Geometry check sheet. Reference: the model listing, model coordinates, mm. A direction names the side the tool comes from. Round coordinates to 2 decimals unless told otherwise and drop trailing zeros. Order: outer loops, then holes, each group sorted by start corner. A loop starts at its lowest first (then second) coordinate and runs counter-clockwise, first axis right, second up.
```python
from build123d import *

# Parameters (mm, degrees)
ESBO_O1_W                                            = 500
ESBO_O1_H                                            = 200
RESSALTO_EXTRUS_O1_DEPTH                             = 40
REBAIXO_PARA_PARAFUSO_ALLEN_SEXTAVADO_DE_D           = 11
REBAIXO_PARA_PARAFUSO_ALLEN_SEXTAVADO_DE_DEPTH       = 40
REBAIXO_PARA_PARAFUSO_ALLEN_SEXTAVADO_DE_CBORE_D     = 18
REBAIXO_PARA_PARAFUSO_ALLEN_SEXTAVADO_DE_CBORE_DEPTH = 7.1
FURO_ROSCADO_DE_M18X2_0_D                            = 16
FURO_ROSCADO_DE_M18X2_0_DEPTH                        = 40


with BuildPart() as part:
    # Esboço1 → Ressalto-extrusão1 (new body)
    with BuildSketch(Plane(origin=(0, 0, 0), x_dir=(1, 0, 0), z_dir=(0, 1, 0))):
        Rectangle(ESBO_O1_W, ESBO_O1_H)
    extrude(amount=RESSALTO_EXTRUS_O1_DEPTH)

    # Rebaixo para parafuso Allen sextavado de M101
    with Locations(Plane(origin=(0, 40, 0), x_dir=(1, 0, 0), z_dir=(0, 1, 0))):
        with Locations((-225, 75), (-75, 75), (75, 75), (-75, -75), (75, -75), (-225, -75), (225, 75), (225, -75)):
            CounterBoreHole(REBAIXO_PARA_PARAFUSO_ALLEN_SEXTAVADO_DE_D / 2, REBAIXO_PARA_PARAFUSO_ALLEN_SEXTAVADO_DE_CBORE_D / 2, REBAIXO_PARA_PARAFUSO_ALLEN_SEXTAVADO_DE_CBORE_DEPTH, depth=REBAIXO_PARA_PARAFUSO_ALLEN_SEXTAVADO_DE_DEPTH)

    # Furo roscado de M18x2.0
    with Locations(Plane(origin=(0, 40, 0), x_dir=(1, 0, 0), z_dir=(0, 1, 0))):
        with Locations((-150, 0), (0, 0), (150, 0)):
            Hole(FURO_ROSCADO_DE_M18X2_0_D / 2, depth=FURO_ROSCADO_DE_M18X2_0_DEPTH)


solid = part.part
```
(1) Material ranges on line 1 (Z direction, x = -225, y = 16); line 2 (X direction, y = 23, z = 75); line 3 (X direction, y = 35, z = 75), recorded low to high.
Returned:
line 1: z = -100 to -80.5, -69.5 to 69.5, 80.5 to 100
line 2: x = -250 to -230.5, -219.5 to -80.5, -69.5 to 69.5, 80.5 to 219.5, 230.5 to 250
line 3: x = -250 to -234, -216 to -84, -66 to 66, 84 to 216, 234 to 250
(2) Set-up check for faces 1 (the flat face through (221, 32.9, -71)), 2 (the cylindrical face through (1.73, 19.72, 7.81)): record each of +Z, -Z, +X, -X, +Y, -Y from which the full face is reachable in a straight line by a thin tool's end or side.
Returned:
face 1: +Y
face 2: +Y, -Y
(3) Sectioned sample at B-B, the plane x = 225. Record the cut outline in (y, z).
Returned:
outline: (0, -100) - (40, -100) - (40, -84) - (32.9, -84) - (32.9, -80.5) - (0, -80.5) - close; (0, -69.5) - (32.9, -69.5) - (32.9, -66) - (40, -66) - (40, 66) - (32.9, 66) - (32.9, 69.5) - (0, 69.5) - close; (0, 80.5) - (32.9, 80.5) - (32.9, 84) - (40, 84) - (40, 100) - (0, 100) - close
(4) Sectioned sample at A-A, the plane x = 0. Record the cut outline in (y, z), and give its area (3 significant figures).
Returned:
outline: (0, -100) - (40, -100) - (40, -8) - (0, -8) - close; (0, 8) - (40, 8) - (40, 100) - (0, 100) - close
area: 7,360 mm2
(5) Depth check by flat-ended pin: P1, Ø1, axis at x = -156, z = -30, coming from the -Y side; P2, Ø12.5, axis at x = 225, z = 75, coming from the +Y side. Enter the tip coordinate at first touch or a pass-through.
Returned:
P1: stops at y = 0
P2: stops at y = 32.9
(6) Sectioned sample at C-C, the plane z = -75. Give the number of separate pieces and of enclosed holes in the cut face, and give its area (3 significant figures).
Returned:
separate pieces: 5
enclosed holes: 0
area: 18,000 mm2
